from build123d import *

# Parameters (mm, degrees)
F1_DEPTH = 18


with BuildPart() as f1:
    # F0 (on Front) → F1 (new body)
    with BuildSketch(Plane.XZ):
        with BuildLine():
            Line((0, 343), (0, 0))
            Line((0, 0), (82, 0))
            Line((82, 0), (82, 275))
            ThreePointArc((82, 275), (96.644661, 310.355339), (132, 325))
            Line((132, 325), (632, 325))
            ThreePointArc((632, 325), (667.355339, 310.355339), (682, 275))
            Line((682, 275), (682, 0))
            Line((682, 0), (764, 0))
            Line((764, 0), (764, 343))
            Line((764, 343), (0, 343))
        make_face()
    extrude(amount=F1_DEPTH)


solid = f1.part
Source: CAD feature listing. Evaluate the final solid. Frame: model axes, mm. A direction names the side the tool comes from. Round coordinates to 2 decimals unless told otherwise and drop trailing zeros. Order: outer loops, then holes, each group sorted by start corner. A loop starts at its lowest first (then second) coordinate and runs counter-clockwise, first axis right, second up. Notation, with made-up numbers: (-7.75, 53.5) - (13.25, 53.5) arc R18 cw to (13.25, 71.5) - close; hole circle Ø11 at (-12, 10.25). An arc over 180 degrees is marked (long way). Use a Markdown table: item, result. Add a question column.
1. Set-up query: faces 1 (the flat face through (764, -9, 169)), 2 (the flat face through (378, -9, 325)). Return all of +Z, -Z, +X, -X, +Y, -Y with unobstructed straight access to the full face (end or side cutting, diameter ignored); none if empty.
2. Section query D-D (x = 122). Return the cut outline in (y, z), then the cut area to 3 significant figures.
3. Section query B-B (y = -7.5). Return the cut outline in (x, z).
4. Section query C-C (x = 395.5). Return the cut outline in (y, z).
5. Line query: probe 1 along X at (y, z) = (-12.5, 147.5); probe 2 along Z at (x, y) = (318.5, -4.5); probe 3 along X at (y, z) = (-7.25, 306). Output: solid intervals per line, ascending.
6. First-contact query: pin 1 (2 mm diameter, centred on x = 315, y = -6.5, fed in from -Z). Flat tip, straight axial feed; report the tip coordinate or a pass-through.
7. Section query A-A (z = 172). Return the cut outline in (x, y).
Derived:
| question | item | result |
|---|---|---|
| 1 | face 1 | +Z, -Z, +X, +Y, -Y |
| 1 | face 2 | -Z, +Y, -Y |
| 2 | outline | (-18, 323.99) - (0, 323.99) - (0, 343) - (-18, 343) - close |
| 2 | area | 342 mm2 |
| 3 | outline | (0, 0) - (82, 0) - (82, 275) arc R50 cw to (132, 325) - (632, 325) arc R50 cw to (682, 275) - (682, 0) - (764, 0) - (764, 343) - (0, 343) - close |
| 4 | outline | (-18, 325) - (0, 325) - (0, 343) - (-18, 343) - close |
| 5 | probe 1 | 0 to 82, 682 to 764 |
| 5 | probe 2 | 325 to 343 |
| 5 | probe 3 | 0 to 92.77, 671.23 to 764 |
| 6 | pin 1 | z = 325 |
| 7 | outline | (0, -18) - (82, -18) - (82, 0) - (0, 0) - close; (682, -18) - (764, -18) - (764, 0) - (682, 0) - close |
